Design review of the part built by this model. Coordinates are the model's own, in mm. A direction names the side the tool comes from. Round coordinates to 2 decimals unless told otherwise and drop trailing zeros. Order: outer loops, then holes, each group sorted by start corner. A loop starts at its lowest first (then second) coordinate and runs counter-clockwise, first axis right, second up. Notation, with made-up numbers: (37.5, -32) - (66.5, -32) arc R30 cw to (66.5, 5) - close; hole circle Ø10 at (53, -31). An arc over 180 degrees is marked (long way). Write item = value, one per line.
Autodesk Inventor part; units mm, degrees
ref_plane "YZ Plane" through (0, 0, 0) normal (1, 0, 0) x (0, 1, 0)
ref_plane "XZ Plane" through (0, 0, 0) normal (0, 1, 0) x (-1, 0, 0)
ref_plane "XY Plane" through (0, 0, 0) normal (0, 0, 1) x (1, 0, 0)
sketch "Boceto1" plane through (0, 0, 0) normal (0, 1, 0) x (-1, 0, 0)
  line L0 (100, 80) -> (-100, 80)
  line L1 (-100, 80) -> (-100, -80)
  line L2 (-100, -80) -> (100, -80)
  line L3 (100, -80) -> (100, 80)
  line L4 (100, 80) -> (-100, -80) construction
  line L5 (-100, 80) -> (100, -80) construction
  point P0 (0, 0)
  dimension "d0" = 200
  dimension "d1" = 160
extrude "Extrusión1" add sketch "Boceto1" along normal blind 20
sketch "Boceto2" plane through (0, 20, 0) normal (0, 1, 0) x (1, 0, 0)
  line L0 (-100, 80) -> (-100, -80)
  line L1 (-100, 80) -> (-70, 80)
  line L2 (-70, 80) -> (-70, 40)
  line L3 (-70, 40) -> (-100, 40)
  line L4 (-100, 40) -> (-100, 80)
  line L5 (100, 80) -> (-100, 80)
  line L6 (0, 80) -> (0, 40)
  line L7 (100, 80) -> (70, 80)
  line L8 (70, 80) -> (70, 40)
  line L9 (70, 40) -> (100, 40)
  line L10 (100, 40) -> (100, 80)
  point P0 (0, 0)
  dimension "d4" = 30
  dimension "d5" = 40
extrude "Extrusión2" cut sketch "Boceto2" against normal blind 10
sketch "Boceto3" plane through (0, 20, 0) normal (0, 1, 0) x (1, 0, 0)
  line L0 (-70, 80) -> (-70, 40)
  line L1 (-70, 80.0001) -> (-70, 40)
  line L2 (-70, 40) -> (-100, 40)
  line L3 (-100, 40) -> (-100, 80.0001)
  line L4 (-100, 40) -> (-70, 40)
  line L5 (-70, 40) -> (-70, 80)
  line L6 (-70, 80) -> (-100, 80)
  line L7 (-100, 80) -> (-100, 40)
  circle A0 centre (-88.25, 58.25) radius 1.75
  circle A1 centre (-81.75, 51.75) radius 1.75
  line L8 (100, 80) -> (-100, 80)
  line L9 (0, 80) -> (0, 56.5)
  circle A2 centre (88.25, 58.25) radius 1.75
  circle A3 centre (81.75, 51.75) radius 1.75
  point P0 (0, 0)
  point P1 (-64.3507, 80)
  point P2 (-74.3507, 0)
  point P3 (-85, 80)
  dimension "d23" = 21.75
  dimension "d24" = 11.75
  dimension "d26" = 11.75
hole "Agujero1" at (-81.75, 20, -51.75) at (-88.25, 20, -58.25) at (81.75, 20, -51.75) at (88.25, 20, -58.25) direction (0, -1, 0) diameter 3.5 end through all
sketch "Boceto4" plane through (-100, 0, 80) normal (0, 0, 1) x (1, 0, 0)
  line L0 (30, 20) -> (60, 20)
  line L1 (60, 20) -> (60, 10)
  line L2 (60, 10) -> (30, 10)
  line L3 (30, 10) -> (30, 20)
  line L4 (0, 0) -> (0, 20)
  line L5 (100, 0) -> (100, 10)
  line L6 (170, 20) -> (140, 20)
  line L7 (140, 20) -> (140, 10)
  line L8 (140, 10) -> (170, 10)
  line L9 (170, 10) -> (170, 20)
  dimension "d34" = 30
  dimension "d35" = 10
  dimension "d36" = 30
extrude "Extrusión3" add sketch "Boceto4" along normal blind 40
sketch "Boceto5" plane through (0, 20, 0) normal (0, 1, 0) x (1, 0, 0)
  line L0 (59.9999, -50) -> (69.9999, -50)
  line L1 (49.9999, -101.75) -> (49.9999, -79.9497)
  line L2 (59.9999, -108.25) -> (59.9999, -50)
  line L3 (40, -80) -> (69.9999, -80)
  line L4 (49.9999, -79.9497) -> (40, -80)
  circle A0 centre (51.7499, -101.75) radius 1.75
  circle A1 centre (58.2499, -108.25) radius 1.75
  line L5 (69.9999, -80) -> (69.9999, -120)
  line L6 (40, -120) -> (40, -80)
  line L7 (69.9999, -120) -> (40, -120)
  line L8 (0, -50) -> (0, -71.75)
  line L9 (-40, -120) -> (-40, -80)
  line L10 (-49.9999, -101.75) -> (-49.9999, -79.9497)
  circle A2 centre (-51.7499, -101.75) radius 1.75
  circle A3 centre (-58.2499, -108.25) radius 1.75
  line L11 (-40, -80) -> (-69.9999, -80)
  line L12 (-69.9999, -120) -> (-40, -120)
  line L13 (-69.9999, -80) -> (-69.9999, -120)
  line L14 (-59.9999, -108.25) -> (-59.9999, -50)
  line L15 (-40, -120) -> (-69.9999, -120)
  line L16 (-69.9999, -80) -> (-69.9999, -120)
  line L17 (-40, -120) -> (-70, -120)
  line L18 (-40, -80) -> (-40, -120)
  line L19 (-59.9999, -110) -> (-49.9999, -110)
  line L20 (-49.9999, -110) -> (-49.9999, -100)
  line L21 (-49.9999, -100) -> (-59.9999, -100)
  line L22 (-59.9999, -100) -> (-59.9999, -110)
  line L23 (-100, 40) -> (-100, -80)
  point P0 (0, 0)
  point P1 (-56.75, -68.25)
  point P2 (-63.25, -61.75)
  point P3 (63.25, -61.75)
  point P4 (56.75, -68.25)
  dimension "d45" = 3.5
  dimension "d46" = 3.5
  dimension "d39" = 10
  dimension "d40" = 10
  dimension "d41" = 40
  dimension "d42" = 0
  dimension "d43" = 6.5
  dimension "d44" = 6.5
  dimension "d47" = 11.7499
  dimension "d48" = 11.75
  dimension "d49" = 0
  dimension "d50" = 11.75
  dimension "d51" = 0
  dimension "d97" = 40.0001
hole "Agujero2" at (-58.2499, 20, 108.25) at (-51.7499, 20, 101.75) at (51.7499, 20, 101.75) at (58.2499, 20, 108.25) direction (0, -1, 0) diameter 3.5 end through all
sketch "Boceto6" plane through (0, 20, 0) normal (0, 1, 0) x (1, 0, 0)
  circle A0 centre (-60.569, -13.1067) radius 10
  circle A1 centre (-29.569, -59.1067) radius 3.5
  line L0 (-60.569, -13.1067) -> (-39.0083, -13.1067)
  circle A2 centre (-29.569, 25.8933) radius 3.5
  circle A3 centre (-88.569, 25.8933) radius 3.5
  circle A4 centre (-88.569, -59.1067) radius 3.5
  line L1 (70.4544, -63.0517) -> (18.4544, -63.0517)
  line L2 (18.4544, -63.0517) -> (18.4544, 6.9483)
  line L3 (18.4544, 6.9483) -> (70.4544, 6.9483)
  line L4 (70.4544, 6.9483) -> (70.4544, -63.0517)
  line L5 (70.4544, 6.9483) -> (48.4544, 6.9483)
  line L6 (48.4544, 6.9483) -> (48.4544, 48.9483)
  line L7 (48.4544, 48.9483) -> (70.4544, 48.9483)
  line L8 (70.4544, 48.9483) -> (70.4544, 6.9483)
  line L9 (77.2288, -8.158) -> (77.2281, -5.6604)
  circle A5 centre (63.7706, -5.7606) radius 1.75
  line L10 (70.7641, -24.1464) -> (70.7641, 22.2796)
  circle A6 centre (35.8307, -5.7609) radius 1.75
  line L11 (25.1581, -13.2381) -> (25.1581, -10.7404)
  circle A7 centre (68.8507, -57.8309) radius 1.75
  line L12 (26.4277, 35.0051) -> (26.4277, 37.5029)
  circle A8 centre (20.6074, -56.5614) radius 1.75
  line L13 (18.6941, -55.9176) -> (70.7641, -55.9176)
  line L14 (18.6941, -55.9176) -> (18.6941, -7.6743)
  line L15 (44.7291, -55.9176) -> (44.7291, -31.7959)
  line L16 (63.7706, -28.0517) -> (26.4277, -28.0517)
  line L17 (44.7291, -23.5247) -> (44.7291, -31.7959)
  point P0 (0, 0)
  point P1 (-60.569, -16.6067)
  point P2 (45.425, 12.8886)
  point P3 (44.7291, -28.0517)
  dimension "d59" = 7
  dimension "d60" = 7
  dimension "d61" = 7
  dimension "d62" = 39
  dimension "d63" = 46
  dimension "d64" = 59
  dimension "d65" = 46
  dimension "d66" = 39
  dimension "d67" = 59
  dimension "d68" = 52
  dimension "d69" = 70
  dimension "d70" = 22
  dimension "d71" = 42
  dimension "d72" = 3.5
  dimension "d73" = 3.5
  dimension "d74" = 3.5
  dimension "d75" = 3.5
  dimension "d142" = 17.3763
  dimension "d143" = 12.7092
  dimension "d144" = 6.6837
  dimension "d145" = 12.7089
  dimension "d146" = 5.2208
  dimension "d147" = 1.6037
  dimension "d148" = 2.1531
  dimension "d149" = 6.4903
hole "Agujero3" at (68.8507, 20, 57.8309) at (20.6074, 20, 56.5614) at (63.7706, 20, 5.7606) at (35.8307, 20, 5.7609) direction (0, -1, 0) diameter 3.5 end through all
sketch "Boceto7" plane through (0, 20, 0) normal (0, 1, 0) x (1, 0, 0)
  circle A0 centre (-60.569, -13.1067) radius 10
  circle A1 centre (-29.569, -59.1067) radius 3.5
  line L0 (-60.569, -13.1067) -> (-39.0083, -13.1067)
  circle A2 centre (-29.569, 25.8933) radius 3.5
  circle A3 centre (-88.569, 25.8933) radius 3.5
  circle A4 centre (-88.569, -59.1067) radius 3.5
  point P0 (0, 0)
  point P1 (-60.569, -16.6067)
  dimension "d83" = 7
  dimension "d84" = 7
  dimension "d85" = 7
  dimension "d86" = 39
  dimension "d87" = 46
  dimension "d88" = 59
  dimension "d89" = 46
  dimension "d90" = 39
  dimension "d91" = 59
extrude "Extrusión4" cut sketch "Boceto7" against normal blind 20
ref_plane "Plano de trabajo1" through (0, 0, -80) normal (-1, 0, 0) x (0, 0, 1)
ref_plane "Plano de trabajo2" through (100, 0, 0) normal (0, 0, -1) x (-1, 0, 0)
sketch "Boceto8" plane through (0, 20, 0) normal (0, 1, 0) x (1, 0, 0)
  line L0 (80, -15) -> (90, -15)
  circle A0 centre (85, -10) radius 1.75
  line L1 (85, 10) -> (85, -10)
  line L2 (90, -15) -> (90, 15)
  circle A1 centre (85, 10) radius 1.75
  line L3 (80, 15) -> (80, -15)
  line L4 (90, 15) -> (80, -15) construction
  line L5 (80, 15) -> (90, -15) construction
  line L6 (90, 15) -> (80, 15)
  line L7 (100, -80) -> (100, 40)
  line L8 (0, 0) -> (20, -20)
  line L9 (0, 0) -> (28.2843, 0) construction
  line L10 (15, -60) -> (15, -70)
  circle A2 centre (10, -65) radius 1.75
  line L11 (-10, -65) -> (10, -65)
  line L12 (15, -70) -> (-15, -70)
  circle A3 centre (-10, -65) radius 1.75
  line L13 (-15, -60) -> (15, -60)
  line L14 (-15, -70) -> (15, -60) construction
  line L15 (-15, -60) -> (15, -70) construction
  line L16 (-15, -70) -> (-15, -60)
  line L17 (0, 0) -> (18.6615, 18.6615)
  line L18 (0, 0) -> (26.3913, 0) construction
  line L19 (-15, 60) -> (-15, 70)
  circle A4 centre (-10, 65) radius 1.75
  line L20 (10, 65) -> (-10, 65)
  line L21 (-15, 70) -> (15, 70)
  circle A5 centre (10, 65) radius 1.75
  line L22 (15, 60) -> (-15, 60)
  line L23 (15, 70) -> (-15, 60) construction
  line L24 (15, 60) -> (-15, 70) construction
  line L25 (15, 70) -> (15, 60)
  line L26 (70, 80) -> (-70, 80)
  line L27 (-40, -80) -> (40, -80)
  point P0 (86.9608, 0)
  point P1 (86.9608, 0)
  point P2 (85, 15)
  point P3 (0, -69.1269)
  point P4 (0, -69.1269)
  point P5 (-15, -67.1661)
  point P6 (0, 69.7066)
  point P7 (0, 69.7066)
  point P8 (15, 67.7458)
  point P9 (-15, 65)
  point P10 (15, -65)
  dimension "d98" = 10
  dimension "d99" = 30
  dimension "d100" = 10
  dimension "d101" = 5
  dimension "d102" = 5
  dimension "d103" = 5
  dimension "d104" = 5
  dimension "d105" = 45
  dimension "d106" = 45
  dimension "d107" = 10
  dimension "d108" = 10
  dimension "d109" = 30
  dimension "d110" = 5
  dimension "d111" = 5
  dimension "d112" = 5
  dimension "d113" = 5
  dimension "d114" = 10
  dimension "d115" = 30
  dimension "d116" = 5
  dimension "d117" = 5
  dimension "d118" = 5
  dimension "d119" = 5
  dimension "d120" = 10
hole "Agujero4" at (-10, 20, -65) at (10, 20, -65) at (85, 20, -10) at (85, 20, 10) at (10, 20, 65) at (-10, 20, 65) direction (0, -1, 0) diameter 3.5 end through all
sketch "Boceto9" plane through (0, 20, 0) normal (0, 1, 0) x (1, 0, 0)
  circle A0 centre (10, -10) radius 1.75
  line L0 (6.803, 0) -> (14.6069, 0)
  line L1 (0, 0) -> (0, -4.8284)
  line L2 (0, 0) -> (20.0354, 0)
  circle A1 centre (10, 10) radius 1.75
  line L3 (0, 0) -> (0, 4.8284)
  circle A2 centre (-10, 10) radius 1.75
  circle A3 centre (-10, -10) radius 1.75
  dimension "d128" = 3.5
  dimension "d129" = 10
  dimension "d130" = 10
hole "Agujero5" at (-10, 20, 10) at (-10, 20, -10) at (10, 20, -10) at (10, 20, 10) direction (0, -1, 0) diameter 3.5 end through all
sketch "Boceto10" plane through (0, 0, 0) normal (0, -1, 0) x (1, 0, 0)
  line L0 (-16, 16) -> (16, 16)
  line L1 (16, 16) -> (16, -16)
  line L2 (16, -16) -> (-16, -16)
  line L3 (-16, -16) -> (-16, 16)
  line L4 (-16, 16) -> (16, -16) construction
  line L5 (16, 16) -> (-16, -16) construction
  point P0 (0, 0)
  point P1 (0, 0)
  dimension "d138" = 32
  dimension "d139" = 32
extrude "Extrusión5" cut sketch "Boceto10" against normal blind 10
split "Dividir1" plane through (100, 0, 0) removes the side toward (0, 0, 1)
split "Dividir2" plane through (0, 0, -80) removes the side toward (-1, 0, 0)
properties part number "base_mid_2"
Item 1: The part is to be moulded in two halves that separate along X. For faces 4 (the face through (70, 15, -60)), 5 (the face through (8, 5, -16)), 6 (the face through (88.92, 4.93, -56.633)), say which applies: +X half, -X half, draft (parallel to the pull), parting line (faces both ways), or undercut.
Data:
face_4 = +X half
face_5 = draft
face_6 = undercut
Item 2: Take a section at D-D, the plane x = 10. State the section outline as (y, z) points.
Data:
outline = (0, -80) - (20, -80) - (20, -66.75) - (0, -66.75) - close; (0, -63.25) - (20, -63.25) - (20, -11.75) - (10, -11.75) - (10, -16) - (0, -16) - close; (10, -8.25) - (20, -8.25) - (20, 0) - (10, 0) - close
Item 3: Take a section at A-A, the plane x = 88.25. State the section outline as (y, z) points.
Data:
outline = (0, -80) - (10, -80) - (10, -60) - (0, -60) - close; (0, -56.5) - (10, -56.5) - (10, -40) - (20, -40) - (20, 0) - (0, 0) - close
Item 4: For line 1 along X through (y, z) = (13, -10); line 2 along X through (y, z) = (4, -65); line 3 along Z through (x, y) = (81.75, 2.75), list the stretches that pass through material, from the lowest coordinate up. Write a range as [from, to].
Data:
line_1 = [0, 8.25], [11.75, 83.25], [86.75, 100]
line_2 = [0, 8.25], [11.75, 100]
line_3 = [-80, -53.5], [-50, 0]
Item 5: Take a section at C-C, the plane y = 2.25. State the section outline as (x, z) points, and give its area (3 significant figures).
Data:
outline = (0, -80) - (100, -80) - (100, 0) - (16, 0) - (16, -16) - (0, -16) - close; hole circle Ø3.5 at (10, -65); hole circle Ø3.5 at (81.75, -51.75); hole circle Ø3.5 at (85, -10); hole circle Ø3.5 at (88.25, -58.25)
area = 7,710 mm2
Item 6: For faces 1 (the face through (85, 15, -40)), 2 (the face through (8, 10, -8)), 3 (the face through (51, 0, -39)), list the 3-axis set-ups (+Z, -Z, +X, -X, +Y, -Y) from which the entire face can be reached by the end or side of a thin tool; tool diameter is ignored.
Data:
face_1 = -Z, +X, +Y
face_2 = +Z, -X, -Y
face_3 = +Z, -Z, +X, -X, -Y
Item 7: Insertion check: P1, Ø10, axis at x = 18, z = -39.5, coming from the -Y side; P2, Ø2, axis at x = 10, z = -10, coming from the -Y side; P3, Ø3, axis at x = 89.5, y = 14.5, coming from the -Z side; P4, Ø8, axis at x = 8.5, y = 5, coming from the +Z side. Each pin has a flat end and moves straight along its axis. Give the tip position at first contact, or say it passes through.
Data:
P1 = 0
P2 = through
P3 = -40
P4 = -16
Item 8: Take a section at B-B, the plane z = -10. State the section outline as (x, y) points, and give its area (4 significant figures).
Data:
outline = (0, 10) - (8.25, 10) - (8.25, 20) - (0, 20) - close; (11.75, 10) - (16, 10) - (16, 0) - (83.25, 0) - (83.25, 20) - (11.75, 20) - close; (86.75, 0) - (100, 0) - (100, 20) - (86.75, 20) - close
area = 1,735 mm2
